The listing builds one solid part. Answer for the finished solid, in the listing's coordinates (mm). A direction names the side the tool comes from. Coordinates: 2 decimals unless noted, no trailing zeros. Loops run counter-clockwise (first coordinate to the right, second up) from the corner with the lowest first, then second, coordinate; pieces in that order, holes last. Notation, with made-up numbers: (73.5, 69.25) -> (104.5, 69.25) arc R19 ccw to (104.5, 99.25) -> close; hole circle Ø6 at (-17, 70). An arc over 180 degrees is marked (long way). Answer in a Markdown table with one row per item.
Solid Edge part; units mm, degrees
sketch "Sketch1" plane through (0, 0, 0) normal (0, 0, 1) x (1, 0, 0)
  line L0 (-13, -25) -> (13, -25)
  line L1 (13, -25) -> (13, 25)
  line L2 (13, 25) -> (-13, 25)
  line L3 (-13, 25) -> (-13, -25)
  dimension "D1" = 13
  dimension "D2" = 13
extrude "Protrusion1" add sketch "Sketch1" along normal blind 6
sketch "Sketch2" plane through (0, -25, 3) normal (0, -1, 0) x (1, 0, 0)
  line L0 (-5, -3) -> (5, -3)
  line L1 (5, -3) -> (5, -1.7)
  line L2 (5, -1.7) -> (-5, -1.7)
  line L3 (-5, -1.7) -> (-5, -3)
  dimension "D1" = 5
  dimension "D2" = 5
extrude "Cutout1" cut sketch "Sketch2" against normal through all
sketch "Sketch3" plane through (0, 0, 6) normal (0, 0, 1) x (1, 0, 0)
  circle A0 centre (-8, 20) radius 1.7
extrude "Cutout2" cut sketch "Sketch3" against normal through all
mirror "Mirror1" about plane through (0, 0, 0) normal (1, 0, 0) of "Cutout2"
mirror "Mirror2" about plane through (0, 0, 0) normal (0, -1, 0) of "Cutout2", "Mirror1"
sketch "Sketch4" plane through (0, 0, 6) normal (0, 0, 1) x (1, 0, 0)
  line L0 (0.5, -11) -> (1.5, -11)
  line L1 (1.5, -11) -> (1.5, 11)
  line L2 (1.5, 11) -> (0.5, 11)
  line L3 (0.5, 11) -> (0.5, -11)
  dimension "D1" = 1.5
  dimension "D2" = 1.5
extrude "Cutout3" cut sketch "Sketch4" against normal through all
Item 1: A tool of negligible diameter and unlimited length cuts with its end or side. For faces 4 (the face through (5, 0, 1)), 5 (the face through (0.5, 0, 4)), 6 (the face through (13, 0, 3)), from which of +Z, -Z, +X, -X, +Y, -Y can it reach the whole face along a straight path? Write none if from no direction.
Findings below:
| item | result |
|---|---|
| face 4 | -Z, +Y, -Y |
| face 5 | +Z, -Z |
| face 6 | +Z, -Z, +X, +Y, -Y |
Item 2: Find the intervals of material crossed by probe 1 along X at (y, z) = (-20, 2.5); probe 2 along Y at (x, z) = (-8, 3.8); probe 3 along Y at (x, z) = (8.75, 0.65), in increasing order.
Findings below:
| item | result |
|---|---|
| probe 1 | x = -13 to -9.7, -6.3 to 6.3, 9.7 to 13 |
| probe 2 | y = -25 to -21.7, -18.3 to 18.3, 21.7 to 25 |
| probe 3 | y = -25 to -21.53, -18.47 to 18.47, 21.53 to 25 |
Item 3: Flat-ended cylindrical pins translate along their axes: pin 1 Ø5.5 at (x, y) = (8, 20) entering from +Z; pin 2 Ø2 at (x, y) = (8, -20) entering from +Z. Find the tip coordinate at first contact, or state that the pin passes through.
Findings below:
| item | result |
|---|---|
| pin 1 | stops at z = 6 |
| pin 2 | passes through |
Item 4: Determine the mould class of faces 1 (the face through (0, -25, 3)), 2 (the face through (1.5, 0, 4)), 3 (the face through (-13, 0, 3)) for opening direction X: +X half, -X half, draft (parallel to the pull), parting line (faces both ways), or undercut.
Findings below:
| item | result |
|---|---|
| face 1 | draft |
| face 2 | undercut |
| face 3 | -X half |
Item 5: A cutting plane is placed at B-B, the plane z = 2.1. Determine the outline of the cut face in (x, y).
Findings below:
| item | result |
|---|---|
| outline | (-13, -25) -> (13, -25) -> (13, 25) -> (-13, 25) -> close; hole circle Ø3.4 at (-8, -20); hole circle Ø3.4 at (-8, 20); hole (0.5, -11) -> (1.5, -11) -> (1.5, 11) -> (0.5, 11) -> close; hole circle Ø3.4 at (8, -20); hole circle Ø3.4 at (8, 20) |
Item 6: A cutting plane is placed at A-A, the plane y = -1.5. Determine the outline of the cut face in (x, z).
Findings below:
| item | result |
|---|---|
| outline | (-13, 0) -> (-5, 0) -> (-5, 1.3) -> (0.5, 1.3) -> (0.5, 6) -> (-13, 6) -> close; (1.5, 1.3) -> (5, 1.3) -> (5, 0) -> (13, 0) -> (13, 6) -> (1.5, 6) -> close |
Item 7: A cutting plane is placed at C-C, the plane x = -8. Determine the outline of the cut face in (y, z).
Findings below:
| item | result |
|---|---|
| outline | (-25, 0) -> (-21.7, 0) -> (-21.7, 6) -> (-25, 6) -> close; (-18.3, 0) -> (18.3, 0) -> (18.3, 6) -> (-18.3, 6) -> close; (21.7, 0) -> (25, 0) -> (25, 6) -> (21.7, 6) -> close |
Item 8: A cutting plane is placed at D-D, the plane y = -20. Determine the outline of the cut face in (x, z), plus the area to 3 significant figures.
Findings below:
| item | result |
|---|---|
| outline | (-13, 0) -> (-9.7, 0) -> (-9.7, 6) -> (-13, 6) -> close; (-6.3, 0) -> (-5, 0) -> (-5, 1.3) -> (5, 1.3) -> (5, 0) -> (6.3, 0) -> (6.3, 6) -> (-6.3, 6) -> close; (9.7, 0) -> (13, 0) -> (13, 6) -> (9.7, 6) -> close |
| area | 102 mm2 |
